Autodesk Inventor part; units mm, degrees
ref_plane "YZ Plane" through (0, 0, 0) normal (1, 0, 0) x (0, 1, 0)
ref_plane "XZ Plane" through (0, 0, 0) normal (0, 1, 0) x (-1, 0, 0)
ref_plane "XY Plane" through (0, 0, 0) normal (0, 0, 1) x (1, 0, 0)
sketch "Sketch1" plane through (0, 0, 0) normal (0, 1, 0) x (-1, 0, 0)
  circle A0 centre (0, 0) radius 135
  circle A1 centre (0, 0) radius 110
  dimension "d0" = 270
  dimension "d1" = 220
extrude "Extrusion1" add sketch "Sketch1" along normal mid plane 47
sketch "Sketch2" plane through (0, 0, 0) normal (0, 0, 1) x (1, 0, 0)
  circle A0 centre (0, -20.5) radius 18
  line L0 (-135, -23.5) -> (135, -23.5)
  dimension "d4" = 36
  dimension "d38" = 3
extrude "Extrusion2" cut sketch "Sketch2" against normal through all
sketch "Sketch3" plane through (0, 23.5, 0) normal (0, 1, 0) x (1, 0, 0)
  circle A0 centre (0, 0) radius 127.5
  circle A1 centre (-127.5, 0) radius 2
  circle A2 centre (-103.1497, -74.9426) radius 2
  circle A3 centre (-39.3997, -121.2597) radius 2
  circle A4 centre (39.3997, -121.2597) radius 2
  circle A5 centre (103.1497, -74.9426) radius 2
  circle A6 centre (127.5, 0) radius 2
  circle A7 centre (103.1497, 74.9426) radius 2
  circle A8 centre (39.3997, 121.2597) radius 2
  circle A9 centre (-39.3997, 121.2597) radius 2
  circle A10 centre (-103.1497, 74.9426) radius 2
  dimension "d7" = 255
  dimension "d8" = 4
  dimension "d11" = 360
hole "Hole1" at (39.3997, 23.5, 121.2597) at (-39.3997, 23.5, 121.2597) at (-103.1497, 23.5, 74.9426) at (-127.5, 23.5, 0) at (-103.1497, 23.5, -74.9426) at (-39.3997, 23.5, -121.2597) at (39.3997, 23.5, -121.2597) at (103.1497, 23.5, -74.9426) at (127.5, 23.5, 0) at (103.1497, 23.5, 74.9426) direction (0, -1, 0) diameter 5 end through all
sketch "Sketch4" plane through (0, 23.5, 0) normal (0, 1, 0) x (1, 0, 0)
  circle A0 centre (0, 0) radius 140
extrude "Extrusion3" cut sketch "Sketch4" against normal blind 27
sketch "Sketch7" plane through (0, -3.5, 0) normal (0, 1, 0) x (1, 0, 0)
  line L0 (0, 0) -> (70, 0)
  line L1 (80, -100) -> (60, -100)
  line L2 (60, -100) -> (60, 100)
  line L3 (60, 100) -> (80, 100)
  line L4 (80, 100) -> (80, -100)
  line L5 (80, -100) -> (60, 100) construction
  line L6 (60, -100) -> (80, 100) construction
  dimension "d39" = 70
  dimension "d40" = 20
  dimension "d41" = 200
extrude "Extrusion7" cut sketch "Sketch7" against normal blind 15
sketch "Sketch8" plane through (0, -3.5, 0) normal (0, 1, 0) x (1, 0, 0)
  line L0 (-129.4827, -38.1999) -> (129.4827, 38.1999)
  line L1 (0, 134.8703) -> (0, -135)
  arc A0 (-5.9161, 134.8703) -> (5.9161, 134.8703) centre (0, 0) ccw
  arc A1 (5.9161, 134.8703) -> (-5.9161, 134.8703) centre (0, 0) ccw
  point P0 (5.9161, 134.8703)
  point P1 (0, 0)
extrude "Extrusion8" cut sketch "Sketch8" against normal through all contours A0 A1 L0 | L0 L1 A0 picked at (-84.5453, -30.4063)
sketch "Sketch9" plane through (0, -3.5, 110) normal (-1, 0, 0) x (0, 0, 1)
  line L0 (-148.1999, 0) -> (25, 0)
  line L1 (22.5, 0) -> (40, 0)
  line L2 (45, -5) -> (45, -15)
  line L3 (40, -20) -> (22.5, -20)
  line L4 (22.5, -20) -> (22.5, 0)
  line L5 (25, 0) -> (25, -20)
  arc A0 (45, -5) -> (40, 0) centre (40, -5) ccw
  arc A1 (40, -20) -> (45, -15) centre (40, -15) ccw
  point P0 (-110, 3.5)
  point P1 (45, -20)
  point P2 (45, 0)
  point P3 (25, 0)
  dimension "d46" = 22.5
  dimension "d47" = 20
  dimension "d48" = 20
  dimension "d49" = 5
extrude "Extrusion9" add sketch "Sketch9" against normal blind 10
sketch "Sketch10" plane through (105.5044, -23.5, -31.1258) normal (-0.283, 0, -0.9591) x (-0.9591, 0, 0.283)
  line L0 (0, 0) -> (-25, 0)
  line L1 (-22.5, 0) -> (-40, 0)
  line L2 (-45, 5) -> (-45, 15)
  line L3 (-40, 20) -> (-22.5, 20)
  line L4 (-22.5, 20) -> (-22.5, 0)
  line L5 (-25, 0) -> (-25, 20)
  arc A0 (-40, 20) -> (-45, 15) centre (-40, 15) ccw
  arc A1 (-45, 5) -> (-40, 0) centre (-40, 5) ccw
  point P0 (110, 23.5)
  point P1 (-45, 20)
  point P2 (-45, 0)
  point P3 (-25, 0)
  dimension "d52" = 22.5
  dimension "d53" = 20
  dimension "d54" = 20
  dimension "d55" = 5
extrude "Extrusion10" add sketch "Sketch10" against normal blind 10
fillet "Fillet1" radius 2.5 2 edges at (131.9566, -13.5, -28.5036) (10, -13.5, 134.6291)
sketch "Sketch11" plane through (10, -3.5, 110) normal (1, 0, 0) x (0, 0, -1)
  line L0 (-45, -5) -> (-45, -15)
  line L1 (-40, -20) -> (-26.9306, -20)
  point P0 (110, 3.5)
  point P1 (-35, -10)
  dimension "d59" = 10
  dimension "d60" = 10
hole "Hole2" at (10, -13.5, 145) direction (-1, 0, 0) diameter 8.2 end through all counterbore diameter 13.2 counterbore depth 6
sketch "Sketch12" plane through (108.334, -23.5, -21.5345) normal (0.283, 0, 0.9591) x (0.9591, 0, -0.283)
  line L0 (41.6, 7.2662) -> (37.7338, 3.4)
  line L1 (37.7338, 3.4) -> (32.2662, 3.4)
  line L2 (32.2662, 3.4) -> (28.4, 7.2662)
  line L3 (28.4, 7.2662) -> (28.4, 12.7338)
  line L4 (28.4, 12.7338) -> (32.2662, 16.6)
  line L5 (32.2662, 16.6) -> (37.7338, 16.6)
  line L6 (37.7338, 16.6) -> (41.6, 12.7338)
  line L7 (41.6, 12.7338) -> (41.6, 7.2662)
  line L8 (45, 5) -> (45, 15)
  line L9 (26.9306, 0) -> (40, 0)
  point P0 (-110, 23.5)
  point P1 (35, 10)
  dimension "d68" = 10
  dimension "d69" = 10
  dimension "d70" = 13.2
extrude "Extrusion11" cut sketch "Sketch12" against normal blind 6
sketch "Sketch13" plane through (106.6363, -23.5, -27.2893) normal (0.283, 0, 0.9591) x (0.9591, 0, -0.283)
  line L0 (26.9306, 0) -> (40, 0)
  line L1 (45, 5) -> (45, 15)
  point P0 (-110, 23.5)
  point P1 (35, 10)
  dimension "d73" = 10
  dimension "d74" = 10
hole "Hole3" at (140.2059, -13.5, -37.1929) direction (-0.283, 0, -0.9591) diameter 8.2 end through all
properties part number "Cylinder Spacer Bottom_Q3"
Here's how the part is built. I have some questions about the finished solid (model axes, mm). A direction names the side the tool comes from. Round coordinates to 2 decimals unless told otherwise and drop trailing zeros. Write each loop counter-clockwise with the first axis right and the second up, starting at its lowest first coordinate (ties: lowest second). Pieces come first, ordered by that corner, then holes.
1. Suppose I cut it at B-B (z = 0). List the corners of the cut face in (x, y) for me, and give its area (3 significant figures).
2. Suppose I cut it at A-A (z = 145). List the corners of the cut face in (x, y) for me, and give its area (3 significant figures).
3. For faces 1 (the flat face through (80, -11, 88)), 2 (the flat face through (136.616, -18.194, -32.965)), which set-ups out of +Z, -Z, +X, -X, +Y, -Y let a thin tool reach every point of the face, with its end or its side?
4. If we mould it in two halves opening along Z, with no side actions, what happens to faces 3 (the cylindrical face through (1.972, -13.68, 149.096)), 4 (the flat face through (116.144, -13.36, -34.265)), 5 (the cylindrical face through (4.93, -22.07, 153.5)), 6 (the cylindrical face through (39.29, -13.64, 118.762))? For each: released by +Z, released by -Z, zero draft, split by the parting line, or undercut.
5. Will these pins go through, and if not, where does the flat tip stop? pin 1 Ø3 at (x, z) = (39.4, 121.26) entering from +Y; pin 2 Ø10.5 at (y, z) = (-12, 145) entering from +X; pin 3 Ø10 at (y, z) = (-12, -7) entering from +X; pin 4 Ø6 at (x, y) = (87, -5.5) entering from +Z.
6. I need wall thicknesses on L1, parallel to Z at x = 2.8, y = -13.5; L2, parallel to Y at x = 7.4, z = 145; L3, parallel to Z at x = 41, y = -21.25. Which ranges of each line are inside material? Lowest first, please.
7. Suppose I cut it at D-D (z = 106.5). List the corners of the cut face in (x, y) for me, and give its area (3 significant figures).
8. Suppose I cut it at C-C (x = 77). List the corners of the cut face in (y, z) for me, and give its area (3 significant figures).
Answer sheet:
1. outline: (110, -23.5) - (125, -23.5) - (125, -3.5) - (110, -3.5) - close; (130, -23.5) - (135, -23.5) - (135, -3.5) - (130, -3.5) - close
1. area: 400 mm2
2. outline: (0, -23.5) - (10, -23.5) - (10, -20.1) - (4, -20.1) - (4, -17.6) - (0, -17.6) - close; (0, -9.4) - (4, -9.4) - (4, -6.9) - (10, -6.9) - (10, -3.5) - (0, -3.5) - close
2. area: 88.0 mm2
3. face 1: -Z, +Y
3. face 2: none
4. face 3: undercut
4. face 4: released by -Z
4. face 5: released by +Z
4. face 6: undercut
5. pin 1: passes through
5. pin 2: stops at x = 10
5. pin 3: stops at x = 134.99
5. pin 4: stops at z = 105.68
6. L1: z = 109.96 to 140.9, 149.1 to 155
6. L2: y = -23.5 to -20.1, -6.9 to -3.5
6. L3: z = 102.07 to 119.34, 123.18 to 128.62
7. outline: (27.53, -23.5) - (82.96, -23.5) - (82.96, -3.5) - (27.53, -3.5) - close
7. area: 1,110 mm2
8. outline: (-23.5, 78.56) - (-18.5, 78.56) - (-18.5, 100) - (-3.5, 100) - (-3.5, 110.89) - (-23.5, 110.89) - close
8. area: 325 mm2
